```python
from build123d import *

# Parameters (mm, degrees)
SKETCH1_W               = 5.08
SKETCH1_H               = 7.62
CUT_EXTRUDE1_DEPTH      = 20.176579466
CUT_EXTRUDE1_DEPTH_BACK = 20.176579466
SKETCH2_R               = 3.175
CUT_EXTRUDE2_DEPTH      = 6.35
SKETCH3_R               = 3.175
CUT_EXTRUDE3_DEPTH      = 20.176579466
SKETCH4_R               = 13.063866327
SKETCH4_W               = 7.62
SKETCH4_H               = 7.62
CUT_EXTRUDE4_DEPTH      = 2.54


with BuildPart() as part:
    # Sketch1 → Revolve1 (revolve)
    with BuildSketch(Plane.XY, mode=Mode.PRIVATE) as revolve1_sk:
        with BuildLine():
            Line((-5.08, 12.7), (-5.08, 7.62))
            Line((-5.08, 7.62), (0, 7.62))
            Line((0, 7.62), (0, 12.7))
            Line((0, 12.7), (0, 17.78))
            ThreePointArc((0, 17.78), (-3.592102448, 16.292102448), (-5.08, 12.7))
        make_face()
        with Locations((-2.54, 3.81)):
            Rectangle(SKETCH1_W, SKETCH1_H)
    revolve(revolve1_sk.sketch.rotate(Axis((0, 12.7, 0), (0, -1, 0)), 180), axis=Axis((0, 12.7, 0), (0, -1, 0)))

    # Sketch1_3 → Cut-Extrude1 (cut, two sides: drawn at the far end of the back side and taken through both)
    with BuildSketch(Plane.XY.offset(-CUT_EXTRUDE1_DEPTH_BACK)):
        with BuildLine():
            Line((-5.08, 12.7), (-5.08, 7.62))
            Line((-5.08, 7.62), (0, 7.62))
            Line((0, 7.62), (0, 12.7))
            Line((0, 12.7), (0, 17.78))
            ThreePointArc((0, 17.78), (-3.592102448, 16.292102448), (-5.08, 12.7))
        make_face()
    extrude(amount=CUT_EXTRUDE1_DEPTH + CUT_EXTRUDE1_DEPTH_BACK, mode=Mode.SUBTRACT)

    # Sketch2 → Cut-Extrude2 (cut)
    with BuildSketch(Plane.XZ):
        Circle(SKETCH2_R)
    extrude(amount=-CUT_EXTRUDE2_DEPTH, mode=Mode.SUBTRACT)

    # Sketch3 → Cut-Extrude3 (cut, through all)
    with BuildSketch(Plane.ZY):
        with Locations((0, 12.7)):
            Circle(SKETCH3_R)
    extrude(amount=-CUT_EXTRUDE3_DEPTH, mode=Mode.SUBTRACT)

    # Sketch4 → Cut-Extrude4 (cut)
    with BuildSketch(Plane(origin=(0, 0, 0), x_dir=(1, 0, 0), z_dir=(0, 1, 0))):
        Circle(SKETCH4_R)
        Rectangle(SKETCH4_W, SKETCH4_H, mode=Mode.SUBTRACT)
    extrude(amount=CUT_EXTRUDE4_DEPTH, mode=Mode.SUBTRACT)


solid = part.part
```
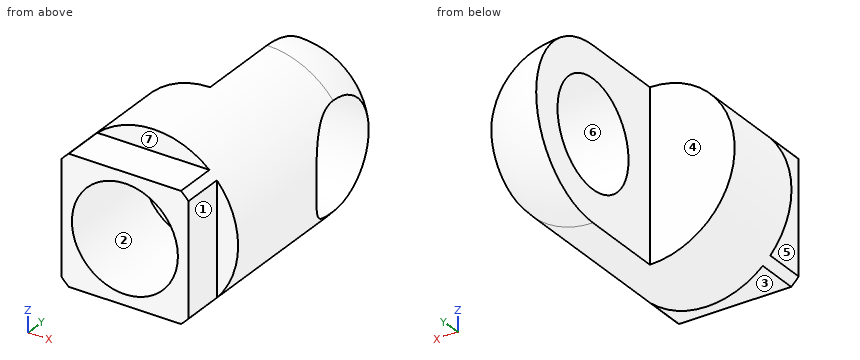
Verification items for the finished model (mm, model axes). Face numbers are marked on the shaded views. A direction names the side the tool comes from. Coordinates: 2 decimals unless noted, no trailing zeros. Loops run counter-clockwise (first coordinate to the right, second up) from the corner with the lowest first, then second, coordinate; pieces in that order, holes last. Notation, with made-up numbers: (-8.5, 76) - (48.5, 76) arc R11 ccw to (48.5, 85) - close; hole circle Ø5 at (-21.75, 46.5). An arc over 180 degrees is marked (long way). Return JSON: item names as keys, results as strings.
1. Go/stop test with flat-tipped pins: pin 1 (1 mm diameter, centred on y = 5.5, z = -3.5, fed in from +X); pin 2 (0.6 mm diameter, centred on x = 0, z = -4.5, fed in from -Y); pin 3 (5 mm diameter, centred on x = 1, z = -3, fed in from +Y); pin 4 (5.5 mm diameter, centred on y = 12.7, z = 0, fed in from +X). Record where each tip stops, or that it passes through.
Established:
{"pin 1": "stops at x = 4.1", "pin 2": "stops at y = 2.54", "pin 3": "stops at y = 17.74", "pin 4": "passes through"}
2. Section check A-A, the plane x = 2. Record the boundary of the cut face in (y, z) (3 decimals), then the cut area to 3 significant figures.
Established:
{"outline": "(0, -3.81) - (2.54, -3.81) - (2.54, -4.67) - (12.7, -4.67) arc R4.67 ccw to (12.7, 4.67) - (2.54, 4.67) - (2.54, 3.81) - (0, 3.81) - (0, 2.466) - (6.35, 2.466) - (6.35, -2.466) - (0, -2.466) - close; hole circle Ø6.35 at (12.7, 0)", "area": "85.5 mm2"}
3. Tool access check on the marked faces 1, 2, 3 and 4. Record the directions out of +Z, -Z, +X, -X, +Y, -Y that give a thin tool (end or side, any length) a straight path to the whole face; none if there is none.
Established:
{"face 1": "+Z, -Z, +X, -Y", "face 2": "-Y", "face 3": "-Z, +X, -X, -Y", "face 4": "+Z, -Z, -X, +Y"}
4. Section check D-D, the plane y = 13.5. Record the boundary of the cut face in (x, z), then the cut area to 3 significant figures.
Established:
{"outline": "(0, -5.02) arc R5.02 ccw to (3.97, -3.07) - (0, -3.07) - close; (0, 3.07) - (3.97, 3.07) arc R5.02 ccw to (0, 5.02) - close", "area": "10.8 mm2"}
5. Section check B-B, the plane y = 5. Record the boundary of the cut face in (x, z) (3 decimals), then the cut area to 3 significant figures.
Established:
{"outline": "circle Ø10.16 at (0, 0); hole circle Ø6.35 at (0, 0)", "area": "49.4 mm2"}
6. Thickness scan on L1, parallel to Z at x = 0, y = 2.5 (3 decimals); L2, parallel to Y at x = -2.5, z = -3.5; L3, parallel to Y at x = -0.75, z = -0.25. Record the ranges inside material, lowest first.
Established:
{"L1": "z = -3.81 to -3.175, 3.175 to 3.81", "L2": "y = 0 to 7.62", "L3": "y = 6.35 to 7.62"}
7. Section check C-C, the plane z = -1. Record the boundary of the cut face in (x, y).
Established:
{"outline": "(-4.98, 2.54) - (-3.81, 2.54) - (-3.81, 0) - (-3.01, 0) - (-3.01, 6.35) - (3.01, 6.35) - (3.01, 0) - (3.81, 0) - (3.81, 2.54) - (4.98, 2.54) - (4.98, 9.69) - (0, 9.69) - (0, 7.62) - (-4.98, 7.62) - close; (0, 15.71) - (3.97, 15.71) arc R4.98 ccw to (0, 17.68) - close"}
8. Mould release check, pull along Y, two halves, no side actions. Record for the marked faces 5, 6 and 7: +Y half, -Y half, draft (parallel to the pull), parting line (faces both ways), or undercut.
Established:
{"face 5": "draft", "face 6": "undercut", "face 7": "-Y half"}
